```python
from build123d import *

# Parameters (mm, degrees)
BOSS_EXTRUDE1_DEPTH = 1.5
SKETCH3_R           = 1.5
SKETCH3_W           = 15.875
SKETCH3_H           = 82.55
CUT_EXTRUDE1_DEPTH  = 144.715413374
FILLET1_R           = 12.7


with BuildPart() as part:
    # Sketch1 → Boss-Extrude1 (new, symmetric)
    with BuildSketch(Plane(origin=(0, 0, 0), x_dir=(1, 0, 0), z_dir=(0, 1, 0))):
        with BuildLine():
            Line((-101.6, 0), (-101.6, 101.6))
            Line((-101.6, 101.6), (101.6, 101.6))
            Line((101.6, 101.6), (101.6, 0))
            add(Edge.make_bspline(
                [(101.6, 0), (101.6, -15.24), (92.836364207, -28.257655975), (72.917051275, -49.879895788), (72.621677222, -76.538397804), (63.5, -101.6)],
                knots=[0, 0, 0, 0, 0.415380003, 0.515380003, 1, 1, 1, 1], degree=3))
            Line((63.5, -101.6), (50.8, -101.6))
            Line((50.8, -101.6), (50.8, -57.15))
            Line((50.8, -57.15), (-50.8, -57.15))
            Line((-50.8, -57.15), (-50.8, -101.6))
            Line((-50.8, -101.6), (-63.5, -101.6))
            add(Edge.make_bspline(
                [(-101.6, 0), (-101.6, -15.24), (-92.836364207, -28.257655975), (-72.917051275, -49.879895788), (-72.621677222, -76.538397804), (-63.5, -101.6)],
                knots=[0, 0, 0, 0, 0.415380003, 0.515380003, 1, 1, 1, 1], degree=3))
        make_face()
    extrude(amount=BOSS_EXTRUDE1_DEPTH, both=True)

    # Sketch3 → Cut-Extrude1 (cut, through all)
    with BuildSketch(Plane(origin=(0, 1.5, 0), x_dir=(1, 0, 0), z_dir=(0, 1, 0))):
        with Locations(Location((-63.499999999, 88.9, 0), (0, 0, 270))):
            Circle(SKETCH3_R)
        with Locations(Location((-73.024999999, -12.7, 0), (0, 0, 270))):
            Circle(SKETCH3_R)
        with Locations(Location((-25.399999999, -47.625, 0), (0, 0, 270))):
            Circle(SKETCH3_R)
        with Locations(Location((25.399999999, -47.625, 0), (0, 0, 90))):
            Circle(SKETCH3_R)
        with Locations(Location((73.024999999, -12.7, 0), (0, 0, 90))):
            Circle(SKETCH3_R)
        with Locations(Location((63.499999999, 88.9, 0), (0, 0, 90))):
            Circle(SKETCH3_R)
        with Locations((-88.9, 50.8)):
            Rectangle(SKETCH3_W, SKETCH3_H)
        with Locations((88.9, 50.8)):
            Rectangle(SKETCH3_W, SKETCH3_H)
    extrude(amount=-CUT_EXTRUDE1_DEPTH, mode=Mode.SUBTRACT)

    # Fillet1
    fillet1_edges = [part.edges().sort_by_distance(p)[0] for p in [
        (101.6, 0, -101.6),
        (-101.6, 0, -101.6),
        (-63.5, -0.75, 101.6),
        (63.5, -0.75, 101.6),
    ]]
    fillet(fillet1_edges, radius=FILLET1_R)


solid = part.part
```
Can you work these out from the model? Positions are in its coordinate system, mm. Coordinates: 2 decimals unless noted, no trailing zeros. Write each loop counter-clockwise with the first axis right and the second up, starting at its lowest first coordinate (ties: lowest second). Pieces come first, ordered by that corner, then holes. Notation, with made-up numbers: (-27.5, 75.5) - (-18.5, 75.5) arc R20 cw to (-18.5, 103.5) - close; hole circle Ø1 at (16, 61). An arc over 180 degrees is marked (long way). Return JSON: item names as keys, results as strings.
Q1. If we section it at B-B (x = -42): Please give me the cut outline in (y, z), then the cut area to 3 significant figures.
Computed values:
{"outline": "(-1.5, -101.6) - (1.5, -101.6) - (1.5, 57.15) - (-1.5, 57.15) - close", "area": "476 mm2"}
Q2. I'm going to push flat-ended pins straight in: pin 1 Ø12 at (x, z) = (-79.5, 47) entering from +Y; pin 2 Ø2.5 at (x, z) = (25.4, 47.625) entering from +Y; pin 3 Ø0.9 at (x, y) = (-88, -0.5) entering from +Z; pin 4 Ø1.5 at (y, z) = (-0.5, 88) entering from +X. Where does each tip first touch, or does it pass through?
Computed values:
{"pin 1": "stops at y = 1.5", "pin 2": "passes through", "pin 3": "stops at z = 33.78", "pin 4": "stops at x = 67.97"}
Q3. Please list where these lines run through material, in increasing order: L1, parallel to X at y = -0.6, z = -88.9; L2, parallel to X at y = -0.85, z = -37.5; L3, parallel to X at y = -0.7, z = 60.5. Write a range as from..to.
Computed values:
{"L1": "x = -101.6..-96.84, -80.96..-65, -62..62, 65..80.96, 96.84..101.6", "L2": "x = -101.6..-96.84, -80.96..80.96, 96.84..101.6", "L3": "x = -74.08..-50.8, 50.8..74.08"}
Q4. If we section it at A-A (z = -85): Please give me the cut outline in (x, y), then the cut area to 3 significant figures.
Computed values:
{"outline": "(-101.6, -1.5) - (-96.84, -1.5) - (-96.84, 1.5) - (-101.6, 1.5) - close; (-80.96, -1.5) - (80.96, -1.5) - (80.96, 1.5) - (-80.96, 1.5) - close; (96.84, -1.5) - (101.6, -1.5) - (101.6, 1.5) - (96.84, 1.5) - close", "area": "514 mm2"}
